```python
from build123d import *

# Parameters (mm, degrees)
CROQUIS1_W              = 97.8
CROQUIS1_H              = 75
CROQUIS1_R              = 1.5
CROQUIS1_R_2            = 3
SALIENTE_EXTRUIR1_DEPTH = 1.5
CROQUIS2_W              = 33.8
CROQUIS2_H              = 5
CORTAR_EXTRUIR1_DEPTH   = 62.696515299
REDONDEO1_R             = 3


with BuildPart() as part:
    # Croquis1 → Saliente-Extruir1 (new, symmetric)
    with BuildSketch(Plane.XY):
        Rectangle(CROQUIS1_W, CROQUIS1_H)
        with Locations((-41.9, 27)):
            Circle(CROQUIS1_R, mode=Mode.SUBTRACT)
        with Locations((-11.9, 27)):
            Circle(CROQUIS1_R, mode=Mode.SUBTRACT)
        with Locations((-11.9, 6.5)):
            Circle(CROQUIS1_R, mode=Mode.SUBTRACT)
        with Locations((-41.9, 6.5)):
            Circle(CROQUIS1_R, mode=Mode.SUBTRACT)
        with Locations((23.1, -10.5)):
            Circle(CROQUIS1_R_2, mode=Mode.SUBTRACT)
        with Locations((23.1, 24.5)):
            Circle(CROQUIS1_R_2, mode=Mode.SUBTRACT)
        with Locations((43.7, -1.75)):
            Circle(CROQUIS1_R, mode=Mode.SUBTRACT)
        with Locations((43.7, -19.25)):
            Circle(CROQUIS1_R, mode=Mode.SUBTRACT)
    extrude(amount=SALIENTE_EXTRUIR1_DEPTH, both=True)

    # Croquis2 → Cortar-Extruir1 (cut, through all)
    with BuildSketch(Plane.XY.offset(1.5)):
        with Locations((0, -35)):
            Rectangle(CROQUIS2_W, CROQUIS2_H)
    extrude(amount=-CORTAR_EXTRUIR1_DEPTH, mode=Mode.SUBTRACT)

    # Redondeo1
    redondeo1_edges = [part.edges().sort_by_distance(p)[0] for p in [
        (16.9, -32.5, 0),
        (-16.9, -32.5, 0),
        (-48.9, 37.5, 0),
        (48.9, 37.5, 0),
    ]]
    fillet(redondeo1_edges, radius=REDONDEO1_R)


solid = part.part
```
The model under review builds one solid part; all positions refer to its coordinate system, in mm. A direction names the side the tool comes from. Coordinates: 2 decimals unless noted, no trailing zeros. Write each loop counter-clockwise with the first axis right and the second up, starting at its lowest first coordinate (ties: lowest second). Pieces come first, ordered by that corner, then holes.
1) We need section C-C on y = -1.75. State the section outline as (x, z) points.
2) We need section A-A on z = -0.9. Count the separate pieces of the cut face and the enclosed holes in it, then the cut area to 3 significant figures.
3) The part is to be moulded in two halves that separate along Y. For faces 3 (the face through (-42.095, 28.487, -0.021)), 4 (the face through (-33, -37.5, 0)), 5 (the face through (-1, 37.5, 0)), say which applies: pulls with the +Y half, pulls with the -Y half, needs draft (parallel to the pull), parting line crosses it, or undercut.
4) Machinability: for faces 1 (the face through (-43.1, 5.6, 0)), 2 (the face through (0, -32.5, 0)), which of the approach directions +Z, -Z, +X, -X, +Y, -Y give a long, thin tool a straight path to every point of the face, cutting with its end or side? Answer none if there is none.
5) We need section D-D on x = -11.9. State the section outline as (y, z) points, then the cut area to 3 significant figures.
6) We need section B-B on x = 23.1. State the section outline as (y, z) points.
7) To check wall thickness, follow probe 1 along Y at (x, z) = (-41.9, -0.8); probe 2 along Y at (x, z) = (23.1, -0.3); probe 3 along Y at (x, z) = (-2.5, -0.65). State the ranges of each line that lie inside material, in increasing order.
Answer list:
1. outline: (-48.9, -1.5) - (42.2, -1.5) - (42.2, 1.5) - (-48.9, 1.5) - close; (45.2, -1.5) - (48.9, -1.5) - (48.9, 1.5) - (45.2, 1.5) - close
2. separate pieces: 1
2. enclosed holes: 8
2. area: 7,070 mm2
3. face 3: undercut
3. face 4: pulls with the -Y half
3. face 5: pulls with the +Y half
4. face 1: +Z, -Z
4. face 2: +Z, -Z, -Y
5. outline: (-32.5, -1.5) - (5, -1.5) - (5, 1.5) - (-32.5, 1.5) - close; (8, -1.5) - (25.5, -1.5) - (25.5, 1.5) - (8, 1.5) - close; (28.5, -1.5) - (37.5, -1.5) - (37.5, 1.5) - (28.5, 1.5) - close
5. area: 192 mm2
6. outline: (-37.5, -1.5) - (-13.5, -1.5) - (-13.5, 1.5) - (-37.5, 1.5) - close; (-7.5, -1.5) - (21.5, -1.5) - (21.5, 1.5) - (-7.5, 1.5) - close; (27.5, -1.5) - (37.5, -1.5) - (37.5, 1.5) - (27.5, 1.5) - close
7. probe 1: y = -37.5 to 5, 8 to 25.5, 28.5 to 37.5
7. probe 2: y = -37.5 to -13.5, -7.5 to 21.5, 27.5 to 37.5
7. probe 3: y = -32.5 to 37.5
